```python
from build123d import *

# Parameters (mm, degrees)
F0_R           = 36.5
F1_DEPTH       = 270
F4_DEPTH       = 30
F4_DEPTH_BACK  = 10
F7_DEPTH       = 10
F7_DEPTH_BACK  = 10
F9_DEPTH       = 230
F10_R          = 37.5
F11_DEPTH      = 50
F13_W          = 135.54436
F13_H          = 40
F14_DEPTH      = 10
F16_W          = 40
F16_H          = 117.55117
F17_DEPTH      = 15
F18_R          = 10
F19_DEPTH      = 10
F20_R          = 10
F21_DEPTH      = 10
F22_W          = 85
F22_H          = 290
F23_DEPTH      = 12
F23_DEPTH_BACK = 2.1


with BuildPart() as f1:
    # F0 (on Front) → F1 (new body)
    with BuildSketch(Plane.XZ):
        Circle(F0_R)
    extrude(amount=F1_DEPTH)

    # F3 (on offset) → F4 (join, two sides)
    with BuildSketch(Plane.XZ.offset(260)) as f4_sk:
        with BuildLine():
            Line((42.5, -36.5), (21.771541, -36.5))
            ThreePointArc((21.771541, -36.5), (0, 42.5), (-21.771541, -36.5))
            Line((-21.771541, -36.5), (-42.5, -36.5))
            Line((-42.5, -36.5), (-42.5, -38.5))
            Line((-42.5, -38.5), (42.5, -38.5))
            Line((42.5, -38.5), (42.5, -36.5))
        make_face()
    extrude(amount=F4_DEPTH)
    extrude(f4_sk.sketch, amount=-F4_DEPTH_BACK)

    # F6 (on offset) → F7 (join, two sides)
    with BuildSketch(Plane.XZ.offset(10)) as f7_sk:
        with BuildLine():
            Line((42.5, -36.5), (21.771541, -36.5))
            ThreePointArc((21.771541, -36.5), (0, 42.5), (-21.771541, -36.5))
            Line((-21.771541, -36.5), (-42.5, -36.5))
            Line((-42.5, -36.5), (-42.5, -38.5))
            Line((-42.5, -38.5), (42.5, -38.5))
            Line((42.5, -38.5), (42.5, -36.5))
        make_face()
    extrude(amount=F7_DEPTH)
    extrude(f7_sk.sketch, amount=-F7_DEPTH_BACK)

    # F8 (on face) → F9 (join, through all)
    with BuildSketch(Plane(origin=(0, -250, 0), x_dir=(-1, 0, 0), z_dir=(0, 1, 0))):
        Polygon((-42.5, -36.5), (-42.5, -38.5), (42.5, -38.5), (42.5, -36.5), (21.771541, -36.5), (0, -37.5), (-21.771541, -36.5), align=None)
    extrude(amount=F9_DEPTH)

    # F10 (on face) → F11 (join)
    with BuildSketch(Plane.XZ.offset(290)):
        Circle(F10_R)
    extrude(amount=F11_DEPTH)

    # F13 (on offset) → F14 (cut)
    with BuildSketch(Plane.XY.offset(46)):
        with Locations((0, -270)):
            Rectangle(F13_W, F13_H)
    extrude(amount=-F14_DEPTH, mode=Mode.SUBTRACT)

    # F16 (on offset) → F17 (cut)
    with BuildSketch(Plane.YZ.offset(-52)):
        with Locations((-270, 0)):
            Rectangle(F16_W, F16_H)
    extrude(amount=F17_DEPTH, mode=Mode.SUBTRACT)

    # F18 (on face) → F19 (join)
    with BuildSketch(Plane.XY.offset(36)):
        with Locations((0, -270)):
            Circle(F18_R)
    extrude(amount=F19_DEPTH)

    # F20 (on face) → F21 (join)
    with BuildSketch(Plane(origin=(-37, 0, 0), x_dir=(0, -1, 0), z_dir=(-1, 0, 0))):
        with Locations((270, 0)):
            Circle(F20_R)
    extrude(amount=F21_DEPTH)

    # F22 (on face) → F23 (join, two sides)
    with BuildSketch(Plane(origin=(0, 0, -38.5), x_dir=(1, 0, 0), z_dir=(0, 0, -1))) as f23_sk:
        with Locations((0, 145)):
            Rectangle(F22_W, F22_H)
    extrude(amount=F23_DEPTH)
    extrude(f23_sk.sketch, amount=-F23_DEPTH_BACK)


solid = f1.part
```
CAD build for the part. Positions are in the model's coordinates, mm. A direction names the side the tool comes from. Coordinates: 2 decimals unless noted, no trailing zeros. Order: outer loops, then holes, each group sorted by start corner. A loop starts at its lowest first (then second) coordinate and runs counter-clockwise, first axis right, second up. Notation, with made-up numbers: (36, -37.75) - (77, -37.75) arc R32 ccw to (77, 0.25) - close; hole circle Ø10 at (-30.5, -12). An arc over 180 degrees is marked (long way). Answer in a Markdown table with one row per item.
1. Slice it at C-C, the plane z = 0. List the corners of the cut face in (x, y).
Answer:
| item | result |
|---|---|
| outline | (-47, -280) - (-37, -280) - (-37, -290) - (-37.5, -290) - (-37.5, -340) - (37.5, -340) - (37.5, -290) - (42.5, -290) - (42.5, -250) - (36.5, -250) - (36.5, -20) - (42.5, -20) - (42.5, 0) - (-42.5, 0) - (-42.5, -20) - (-36.5, -20) - (-36.5, -250) - (-37, -250) - (-37, -260) - (-47, -260) - close |
2. Pull direction Z, two halves, no side cores. Call faces 1 (the face through (-1, 0, -5)), 2 (the face through (-10.4, -269.7, 36)), 3 (the face through (1.567, -133.39, 36.466)): +Z half, -Z half, draft (parallel to the pull), parting line (faces both ways), or undercut.
Answer:
| item | result |
|---|---|
| face 1 | draft |
| face 2 | +Z half |
| face 3 | undercut |
3. Slice it at A-A, the plane x = 32. List the corners of the cut face in (y, z), then the cut area to 3 significant figures.
Answer:
| item | result |
|---|---|
| outline | (-340, -19.55) - (-290, -19.55) - (-290, -27.97) - (-250, -27.97) - (-250, -17.56) - (-20, -17.56) - (-20, -27.97) - (0, -27.97) - (0, 27.97) - (-20, 27.97) - (-20, 17.56) - (-250, 17.56) - (-250, 27.97) - (-290, 27.97) - (-290, 19.55) - (-340, 19.55) - close; (-290, -50.5) - (0, -50.5) - (0, -36.4) - (-290, -36.4) - close |
| area | 17,500 mm² |
4. Slice it at B-B, the plane y = -270. List the corners of the cut face in (x, z), then the cut area to 3 significant figures.
Answer:
| item | result |
|---|---|
| outline | (-47, -10) - (-37, -10) - (-37, -20.91) arc R42.5 ccw to (-21.94, -36.4) - (-42.5, -36.4) - (-42.5, -50.5) - (42.5, -50.5) - (42.5, -36.4) - (21.94, -36.4) arc R42.5 ccw to (22.59, 36) - (10, 36) - (10, 46) - (-10, 46) - (-10, 36) - (-22.59, 36) arc R42.5 ccw to (-37, 20.91) - (-37, 10) - (-47, 10) - close |
| area | 6,740 mm² |
5. Drill centre lines: L1, parallel to Z at x = -14.5, y = -258.5; L2, parallel to Z at x = 6, y = -67; L3, parallel to X at y = -25.5, z = -43.5. Where is each one in solid material? Low to high. Write a range as from..to.
Answer:
| item | result |
|---|---|
| L1 | -50.5..36 |
| L2 | -50.5..-36.4, -36..36 |
| L3 | -42.5..42.5 |
6. Slice it at D-D, the plane x = -18.5. List the corners of the cut face in (y, z), then the cut area to 3 significant figures.
Answer:
| item | result |
|---|---|
| outline | (-340, -32.62) - (-290, -32.62) - (-290, -50.5) - (0, -50.5) - (0, 38.26) - (-20, 38.26) - (-20, 31.46) - (-250, 31.46) - (-250, 36) - (-290, 36) - (-290, 32.62) - (-340, 32.62) - close; hole (-250, -36.4) - (-20, -36.4) - (-20, -31.46) - (-250, -31.46) - close |
| area | 26,200 mm² |
7. 3-axis set-ups, long thin cutter, end or side, ignore diameter. For faces 4 (the face through (-4.88, -314.65, 37.18)), 5 (the face through (-29, -290, 26)), 6 (the face through (37, -250, -3)): which of +Z, -Z, +X, -X, +Y, -Y reach the whole face in a straight line?
Answer:
| item | result |
|---|---|
| face 4 | -Y |
| face 5 | +Z, -X, -Y |
| face 6 | +X |
8. Flat gauge pins, fed straight in: P1, Ø6, axis at y = -110.5, z = 36, coming from the -X side; P2, Ø10, axis at x = -37, y = -191.5, coming from the +Z side; P3, Ø5, axis at x = -8.5, y = -69, coming from the +Z side. Where does each tip first touch, or does it go through?
Answer:
| item | result |
|---|---|
| P1 | x = -15.6 |
| P2 | z = 17.56 |
| P3 | z = 36 |
